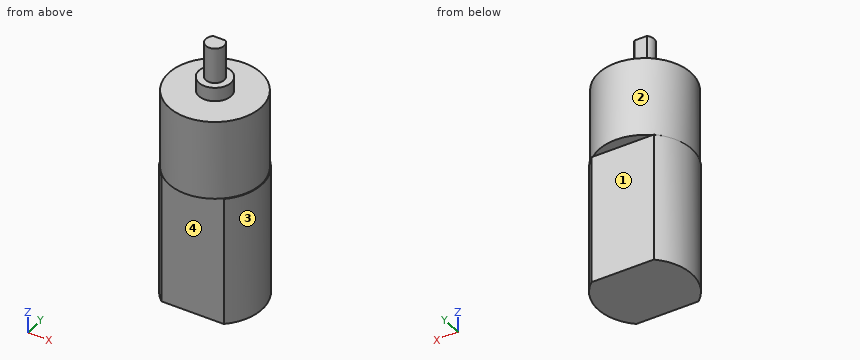
```python
from build123d import *

# Parameters (mm, degrees)
F0_R     = 10
F0_R_2   = 3.5
F1_DEPTH = 17.2
F2_DEPTH = 3
F3_DEPTH = 10.7
F5_DEPTH = 28


with BuildPart() as f1:
    # F0 (on Top) → F1 (new body)
    with BuildSketch(Plane.XY):
        Circle(F0_R)
        Circle(F0_R_2, mode=Mode.SUBTRACT)
        Circle(F0_R_2)
        with BuildLine():
            ThreePointArc((1.3228756555, 1.5), (0, -2), (-1.3228756555, 1.5))
            Line((-1.3228756555, 1.5), (1.3228756555, 1.5))
        make_face(mode=Mode.SUBTRACT)
        with BuildLine():
            Line((1.3228756555, 1.5), (-1.3228756555, 1.5))
            ThreePointArc((-1.3228756555, 1.5), (0, -2), (1.3228756555, 1.5))
        make_face()
    extrude(amount=-F1_DEPTH)

    # F0 (on Top) → F2 (join)
    with BuildSketch(Plane.XY):
        Circle(F0_R_2)
        with BuildLine():
            ThreePointArc((1.3228756555, 1.5), (0, -2), (-1.3228756555, 1.5))
            Line((-1.3228756555, 1.5), (1.3228756555, 1.5))
        make_face(mode=Mode.SUBTRACT)
        with BuildLine():
            Line((1.3228756555, 1.5), (-1.3228756555, 1.5))
            ThreePointArc((-1.3228756555, 1.5), (0, -2), (1.3228756555, 1.5))
        make_face()
    extrude(amount=F2_DEPTH)

    # F0 (on Top) → F3 (join)
    with BuildSketch(Plane.XY):
        with BuildLine():
            Line((1.3228756555, 1.5), (-1.3228756555, 1.5))
            ThreePointArc((-1.3228756555, 1.5), (0, -2), (1.3228756555, 1.5))
        make_face()
    extrude(amount=F3_DEPTH)

    # F4 (on face) → F5 (join)
    with BuildSketch(Plane(origin=(0, 0, -17.2), x_dir=(1, 0, 0), z_dir=(0, 0, -1))):
        with BuildLine():
            ThreePointArc((-6.3804388564, -7.7), (-10, 0), (-6.3804388564, 7.7))
            Line((-6.3804388564, 7.7), (-6.6895440801, 7.7))
            ThreePointArc((-6.6895440801, 7.7), (-10.2, 0), (-6.6895440801, -7.7))
            Line((-6.6895440801, -7.7), (-6.3804388564, -7.7))
        make_face()
        with BuildLine():
            ThreePointArc((10, 0), (9.0499831095, 4.2541515862), (6.3804388564, 7.7))
            Line((6.3804388564, 7.7), (-6.3804388564, 7.7))
            ThreePointArc((-6.3804388564, 7.7), (-10, 0), (-6.3804388564, -7.7))
            Line((-6.3804388564, -7.7), (6.3804388564, -7.7))
            ThreePointArc((6.3804388564, -7.7), (9.0499831095, -4.2541515862), (10, 0))
        make_face()
        with BuildLine():
            ThreePointArc((6.6895440801, -7.7), (10.2, 0), (6.6895440801, 7.7))
            Line((6.6895440801, 7.7), (6.3804388564, 7.7))
            ThreePointArc((6.3804388564, 7.7), (9.0499831095, 4.2541515862), (10, 0))
            ThreePointArc((10, 0), (9.0499831095, -4.2541515862), (6.3804388564, -7.7))
            Line((6.3804388564, -7.7), (6.6895440801, -7.7))
        make_face()
    extrude(amount=F5_DEPTH)


solid = f1.part
```
Can you work these out from the model? Positions are in its coordinate system, mm. Face numbers are marked on the shaded views. A direction names the side the tool comes from. Coordinates: 2 decimals unless noted, no trailing zeros. Loops run counter-clockwise (first coordinate to the right, second up) from the corner with the lowest first, then second, coordinate; pieces in that order, holes last.
1) Imagine slicing it at B-B on y = 0. List the corners of the cut face in (x, z) for me.
2) Imagine slicing it at A-A on x = 0. List the corners of the cut face in (y, z) for me.
3) I need wall thicknesses on probe 1 along Y at (x, z) = (1.25, -30); probe 2 along Z at (x, y) = (-1, -6.75); probe 3 along X at (y, z) = (0, 5). Which ranges of each line are inside material? Lowest first, please.
4) For pin 1 (4 mm diameter, centred on y = 4, z = -6, fed in from +X); pin 2 (4 mm diameter, centred on x = 4.5, z = -13, fed in from -Y); pin 3 (5 mm diameter, centred on y = -3.5, z = -27.5, fed in from +X), each with a flat end and sliding along its axis, tell me the tip position at first contact or that it passes through.
5) Imagine slicing it at D-D on x = -4.25. List the corners of the cut face in (y, z) for me, plus the area to 3 significant figures.
6) Which directions (+Z, -Z, +X, -X, +Y, -Y) give clear straight access to the entire face, cutting with the end or side of a thin tool? Please do the marked faces 1, 2, 3 and 4.
7) Imagine slicing it at C-C on z = 1. List the corners of the cut face in (x, y) for me.
Completed:
1. outline: (-10.2, -45.2) - (10.2, -45.2) - (10.2, -17.2) - (10, -17.2) - (10, 0) - (3.5, 0) - (3.5, 3) - (2, 3) - (2, 10.7) - (-2, 10.7) - (-2, 3) - (-3.5, 3) - (-3.5, 0) - (-10, 0) - (-10, -17.2) - (-10.2, -17.2) - close
2. outline: (-10, -17.2) - (-7.7, -17.2) - (-7.7, -45.2) - (7.7, -45.2) - (7.7, -17.2) - (10, -17.2) - (10, 0) - (3.5, 0) - (3.5, 3) - (1.5, 3) - (1.5, 10.7) - (-2, 10.7) - (-2, 3) - (-3.5, 3) - (-3.5, 0) - (-10, 0) - close
3. probe 1: y = -7.7 to 7.7
3. probe 2: z = -45.2 to 0
3. probe 3: x = -2 to 2
4. pin 1: stops at x = 9.8
4. pin 2: stops at y = -9.68
4. pin 3: stops at x = 10.15
5. outline: (-9.05, -17.2) - (-7.7, -17.2) - (-7.7, -45.2) - (7.7, -45.2) - (7.7, -17.2) - (9.05, -17.2) - (9.05, 0) - (-9.05, 0) - close
5. area: 743 mm2
6. face 1: -Z, +X, -X, +Y
6. face 2: +Z
6. face 3: +Z, -Z, +X
6. face 4: -Z, +X, -X, -Y
7. outline: circle Ø7 at (0, 0)
